Geometry: final body of the model. Coordinates: model frame, mm. Coordinates: 2 decimals unless noted, no trailing zeros. Loops run counter-clockwise (first coordinate to the right, second up) from the corner with the lowest first, then second, coordinate; pieces in that order, holes last. Notation, with made-up numbers: (-34, -4) -> (11, -4) arc R8 ccw to (11, 1) -> close; hole circle Ø7 at (-30, 54). An arc over 180 degrees is marked (long way). One line per item, written item: value. Start each with the question number.
Item 1: Contact query for flat-ended pins moving along their axis: pin 1 Ø8 at (x, y) = (-22.5, -40.5) entering from -Z; pin 2 Ø2 at (x, z) = (-10.5, -2) entering from -Y; pin 3 Ø1.5 at (x, y) = (18.5, -38.5) entering from -Z. Output: stop coordinate, or through.
Item 2: Ray query, probe 1 along Z at (x, y) = (0.5, -27.5); probe 2 along Y at (x, z) = (-23, -22); probe 3 along Y at (x, z) = (-7, -5). Return the intervals inside material, ascending. Write a range as from..to.
Item 3: Section query C-C on z = 0. Return loops of the section in (x, y).
Item 4: Section query D-D on y = -50. Return loops of the section in (x, z), then the cut area to 3 significant figures.
Item 5: Section query B-B on y = -15. Return loops of the section in (x, z).
Item 6: Mould query, pull axis X, two halves, no side actions, for faces 1 (the cylindrical face through (-3.9, -31.6, -17.55)), 2 (the cylindrical face through (-16.989, -43.764, -13.027)), 3 (the flat face through (0, -5.842, 0)), 4 (the flat face through (-1, -31.242, -24)). Classes: +X half, -X half, draft (parallel to the pull), parting line (faces both ways), or undercut.
Item 7: Section query A-A on x = 0. Return loops of the section in (y, z).
from build123d import *

# Parameters (mm, degrees)
F0_W      = 74.656174
F0_H      = 55.025466
F1_DEPTH  = 31.242
F2_R      = 21.408714
F3_DEPTH  = 25.4
F4_R      = 17.978336
F5_DEPTH  = 25.4
F5_FACE_R = 17.978336
F6_DEPTH  = 25.4


with BuildPart() as f1:
    # F0 (on Front) → F1 (new body)
    with BuildSketch(Plane.XZ):
        Rectangle(F0_W, F0_H)
    extrude(amount=F1_DEPTH)

    # F2 (on face) → F3 (join)
    with BuildSketch(Plane.XZ.offset(31.242)):
        Circle(F2_R)
    extrude(amount=F3_DEPTH)

    # F4 (on face) → F5 (cut)
    with BuildSketch(Plane.XZ.offset(56.642)):
        Circle(F4_R)
    extrude(amount=-F5_DEPTH, mode=Mode.SUBTRACT)

    # F5_face (on face) → F6 (cut)
    with BuildSketch(Plane.XZ.offset(31.242)):
        Circle(F5_FACE_R)
    extrude(amount=-F6_DEPTH, mode=Mode.SUBTRACT)


solid = f1.part
Reply:
1. pin 1: stops at z = -10.77
1. pin 2: stops at y = -5.84
1. pin 3: stops at z = -11.97
2. probe 1: z = -27.51..-17.97, 17.97..27.51
2. probe 2: y = -31.24..0
2. probe 3: y = -5.84..0
3. outline: (-37.33, -31.24) -> (-21.41, -31.24) -> (-21.41, -56.64) -> (-17.98, -56.64) -> (-17.98, -5.84) -> (17.98, -5.84) -> (17.98, -56.64) -> (21.41, -56.64) -> (21.41, -31.24) -> (37.33, -31.24) -> (37.33, 0) -> (-37.33, 0) -> close
4. outline: circle Ø42.82 at (0, 0); hole circle Ø35.96 at (0, 0)
4. area: 424 mm²
5. outline: (-37.33, -27.51) -> (37.33, -27.51) -> (37.33, 27.51) -> (-37.33, 27.51) -> close; hole circle Ø35.96 at (0, 0)
6. face 1: undercut
6. face 2: parting line
6. face 3: undercut
6. face 4: draft
7. outline: (-56.64, -21.41) -> (-31.24, -21.41) -> (-31.24, -27.51) -> (0, -27.51) -> (0, 27.51) -> (-31.24, 27.51) -> (-31.24, 21.41) -> (-56.64, 21.41) -> (-56.64, 17.98) -> (-5.84, 17.98) -> (-5.84, -17.98) -> (-56.64, -17.98) -> close
